Verification items for the finished model (mm, model axes). A direction names the side the tool comes from. Round coordinates to 2 decimals unless told otherwise and drop trailing zeros. Order: outer loops, then holes, each group sorted by start corner. A loop starts at its lowest first (then second) coordinate and runs counter-clockwise, first axis right, second up. Notation, with made-up numbers: (27, 31.5) -> (40, 31.5) arc R21 cw to (40, 59.5) -> close; hole circle Ø6 at (-28, 21.25). An arc over 180 degrees is marked (long way). Put each result on its own line as item: value.
from build123d import *

# Parameters (mm, degrees)
SKETCH1_R          = 20.5
SKETCH1_R_2        = 13.5
SKETCH1_R_3        = 1.5875
EXTRUDE1_DEPTH     = 5
CUT_EXTRUDE1_DEPTH = 30.419381367
CIRPATTERN1_COUNT  = 3


with BuildPart() as part:
    # Sketch1 → Extrude1 (new body)
    with BuildSketch(Plane.XY):
        Circle(SKETCH1_R)
        Circle(SKETCH1_R_2, mode=Mode.SUBTRACT)
        with Locations((0, 16.5)):
            Circle(SKETCH1_R_3, mode=Mode.SUBTRACT)
        with Locations((14.289419162, -8.25)):
            Circle(SKETCH1_R_3, mode=Mode.SUBTRACT)
        with Locations((-14.289419162, -8.25)):
            Circle(SKETCH1_R_3, mode=Mode.SUBTRACT)
    extrude(amount=EXTRUDE1_DEPTH)

    # Sketch2 → Cut-Extrude1 (cut, through all)
    with BuildSketch(Plane.XY.offset(5)):
        with BuildLine():
            ThreePointArc((1.5, -16.5), (0, -15), (-1.5, -16.5))
            Line((-1.5, -16.5), (-1.5, -20.4450483))
            ThreePointArc((-1.5, -20.4450483), (0, -20.5), (1.5, -20.4450483))
            Line((1.5, -20.4450483), (1.5, -16.5))
        make_face()
    cut_extrude1 = extrude(amount=-CUT_EXTRUDE1_DEPTH, mode=Mode.SUBTRACT)

    # Sketch4 → Cut-Revolve3 (revolve, cut)
    with BuildSketch(Plane(origin=(0, 0, 0), x_dir=(1, 0, 0), z_dir=(0, 1, 0))):
        Polygon((-13.5, -2.5), (-13.5, -1.5), (-14.5, -2.5), align=None)
        Polygon((-13.5, -3.5), (-13.5, -2.5), (-14.5, -2.5), align=None)
    revolve(axis=Axis((0, 0, 0), (0, 0, 1)), mode=Mode.SUBTRACT)

    # CirPattern1: Cut-Extrude1 ×3 about axis
    cirpattern1_axis = Axis((0, 0, 0), (0, 0, 1))
    for i in range(1, CIRPATTERN1_COUNT):
        add(cut_extrude1.rotate(cirpattern1_axis, i * 360 / CIRPATTERN1_COUNT), mode=Mode.SUBTRACT)


solid = part.part
Item 1: Section check B-B on z = 4.25. State how many separate pieces and enclosed holes the cut face has, then the cut area to 3 significant figures.
Check sheet entries:
separate pieces: 1
enclosed holes: 4
area: 678 mm^2
Item 2: Tool access check on faces 4 (the flat face through (-16.77, 7.95, 2.54)), 5 (the flat face through (1.5, -19, 3)), 6 (the cylindrical face through (17.612, -10.491, 2.465)). Record the directions out of +Z, -Z, +X, -X, +Y, -Y that give a thin tool (end or side, any length) a straight path to the whole face; none if there is none.
Check sheet entries:
face 4: +Z, -Z
face 5: +Z, -Z, -Y
face 6: +Z, -Z, +X
Item 3: Gauge pin test, flat ends, axial feed: pin 1 Ø10 at (x, y) = (-3.5, -1) entering from +Z; pin 2 Ø2 at (y, z) = (-18, 2.5) entering from -X; pin 3 Ø4 at (x, y) = (14.29, -8.25) entering from +Z. Record the tip position at first contact, or that the pin passes through.
Check sheet entries:
pin 1: passes through
pin 2: stops at x = -11.46
pin 3: stops at z = 5
Item 4: Section check D-D on y = 16.5. Record the boundary of the cut face in (x, z).
Check sheet entries:
outline: (-12.17, 0) -> (-1.59, 0) -> (-1.59, 5) -> (-12.17, 5) -> close; (1.59, 0) -> (12.17, 0) -> (12.17, 5) -> (1.59, 5) -> close
Item 5: Section check C-C on x = 0. Record the boundary of the cut face in (y, z), then the cut area to 3 significant figures.
Check sheet entries:
outline: (-15, 0) -> (-13.5, 0) -> (-13.5, 1.5) -> (-14.5, 2.5) -> (-13.5, 3.5) -> (-13.5, 5) -> (-15, 5) -> close; (13.5, 0) -> (14.91, 0) -> (14.91, 5) -> (13.5, 5) -> (13.5, 3.5) -> (14.5, 2.5) -> (13.5, 1.5) -> close; (18.09, 0) -> (20.5, 0) -> (20.5, 5) -> (18.09, 5) -> close
area: 24.6 mm^2
Item 6: Release check for a two-part mould opening along Y. For faces 1 (the flat face through (-14, 0, 5)), 2 (the flat face through (15.27, 10.55, 2.54)), 3 (the cylindrical face through (0.28, 20.5, 2.46)) record: +Y half, -Y half, draft (parallel to the pull), parting line (faces both ways), or undercut.
Check sheet entries:
face 1: draft
face 2: undercut
face 3: +Y half
Item 7: Section check A-A on y = 0. Record the boundary of the cut face in (x, z), then the cut area to 3 significant figures.
Check sheet entries:
outline: (-20.5, 0) -> (-13.5, 0) -> (-13.5, 1.5) -> (-14.5, 2.5) -> (-13.5, 3.5) -> (-13.5, 5) -> (-20.5, 5) -> close; (13.5, 0) -> (20.5, 0) -> (20.5, 5) -> (13.5, 5) -> (13.5, 3.5) -> (14.5, 2.5) -> (13.5, 1.5) -> close
area: 68.0 mm^2
Item 8: Material ranges on L1, parallel to Y at x = 0, z = 0.4; L2, parallel to X at y = 0, z = 4.55; L3, parallel to Y at x = -3, z = 2.2, recorded low to high. Write a range as [from, to].
Check sheet entries:
L1: y = [-15, -13.5], [13.5, 14.91], [18.09, 20.5]
L2: x = [-20.5, -13.5], [13.5, 20.5]
L3: y = [-20.28, -13.88], [13.88, 20.28]
